Verification items for the finished model (mm, model axes). Face numbers are marked on the shaded views. A direction names the side the tool comes from. Coordinates: 2 decimals unless noted, no trailing zeros. Write each loop counter-clockwise with the first axis right and the second up, starting at its lowest first coordinate (ties: lowest second). Pieces come first, ordered by that corner, then holes. Notation, with made-up numbers: (18.25, 19.25) -> (30.25, 19.25) arc R20 ccw to (30.25, 24.25) -> close; hole circle Ø6 at (4, -37.75). An arc over 180 degrees is marked (long way). Use CSV: the item, a comma, the result in double quotes.
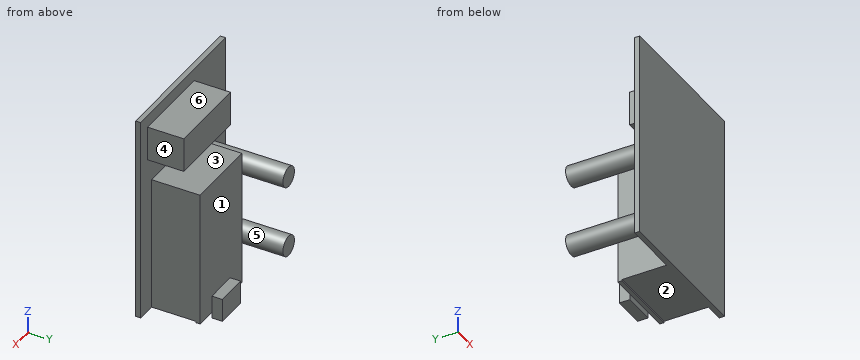
Autodesk Fusion 360 part; units mm, degrees
sketch "Sketch1" plane through (0, 0, 0) normal (0, 1, 0) x (1, 0, 0)
  line L0 (0, 0) -> (37, 0)
  line L1 (37, 0) -> (37, 51)
  line L2 (37, 51) -> (0, 51)
  line L3 (0, 51) -> (0, 0)
  line L4 (13.7, 3) -> (34, 3)
  line L5 (34, 3) -> (34, 11.5)
  line L6 (34, 11.5) -> (13.7, 11.5)
  line L7 (13.7, 11.5) -> (13.7, 3)
  line L8 (14, 17.75) -> (32.25, 17.75)
  line L9 (32.25, 17.75) -> (32.25, 51.35)
  line L10 (32.25, 51.35) -> (14, 51.35)
  line L11 (14, 51.35) -> (14, 17.75)
  line L12 (19.125, 47.15) -> (27.125, 47.15)
  line L13 (27.125, 47.15) -> (27.125, 52.85)
  line L14 (27.125, 52.85) -> (19.125, 52.85)
  line L15 (19.125, 52.85) -> (19.125, 47.15)
  circle A0 centre (9.5, 41.5) radius 2.5
  circle A1 centre (9.5, 23.5) radius 2.5
  dimension "d1" = 37
  dimension "d2" = 51
  dimension "d3" = 3
  dimension "d4" = 3
  dimension "d5" = 20.3
  dimension "d6" = 8.5
  dimension "d7" = 6.25
  dimension "d8" = 18.25
  dimension "d9" = 4.75
  dimension "d10" = 33.6
  dimension "d11" = 5.7
  dimension "d12" = 8
  dimension "d13" = 5.125
  dimension "d15" = 1.5
  dimension "d16" = 9.5
  dimension "d17" = 9.5
  dimension "d18" = 5
  dimension "d19" = 27.5
extrude "Extrude1" add sketch "Sketch1" against normal blind 1.25 contours L0 L1 L2 L3 L8 L9 L11 | L2 L8 L9 L11 L12 L13 L15 | L2 L12 L13 L15 | L4 L5 L6 L7 | A0 | A1
extrude "Extrude2" add sketch "Sketch1" along normal blind 9 contours L4 L5 L6 L7
extrude "Extrude3" add sketch "Sketch1" along normal blind 11 contours L2 L8 L9 L11 L12 L13 L15 | L2 L12 L13 L15
sketch "Sketch3" plane through (0, 11, 0) normal (0, 1, 0) x (-1, 0, 0)
  line L0 (-32.25, -51) -> (-14, -51)
  line L1 (-14, -51) -> (-14, -17.75)
  line L2 (-14, -17.75) -> (-32.25, -17.75)
  line L3 (-32.25, -17.75) -> (-32.25, -51)
  line L4 (-14, -17.75) -> (-32.25, -17.75)
  line L5 (-32.25, -17.75) -> (-32.25, -51.35)
  line L6 (-32.25, -51.35) -> (-14, -51.35)
  line L7 (-14, -51.35) -> (-14, -17.75)
  dimension "d26" = 33.6
  dimension "d27" = 18.25
extrude "Extrude4" add sketch "Sketch3" along normal blind 1
sketch "Sketch4" plane through (0, 12, 0) normal (0, 1, 0) x (-1, 0, 0)
  line L0 (-14, -51.35) -> (-14, -17.75)
  line L1 (-14, -17.75) -> (-32.25, -17.75)
  line L2 (-32.25, -17.75) -> (-32.25, -51.35)
  line L3 (-32.25, -51.35) -> (-14, -51.35)
  line L4 (-19.125, -47.15) -> (-27.125, -47.15)
  line L5 (-27.125, -47.15) -> (-27.125, -52.85)
  line L6 (-27.125, -52.85) -> (-19.125, -52.85)
  line L7 (-19.125, -52.85) -> (-19.125, -47.15)
  line L8 (-32.25, -51.35) -> (-14, -51.35)
  dimension "d30" = 5.125
  dimension "d31" = 8
  dimension "d32" = 5.7
  dimension "d33" = 1.5
extrude "Extrude5" add sketch "Sketch4" along normal blind 2.6 contours L3 L5 L6 L7 L8 | L3 L4 L5 L7 L8
extrude "Extrude6" add sketch "Sketch1" along normal blind 21 contours A0 | A1
sketch "Sketch6" plane through (0, -1.25, 0) normal (0, -1, 0) x (1, 0, 0)
  line L0 (0, 0) -> (0, -51)
  line L1 (0, -51) -> (37, -51)
  line L2 (37, -51) -> (37, 0)
  line L3 (37, 0) -> (0, 0)
  line L4 (4, -4) -> (33, -4)
  line L5 (33, -4) -> (33, -49)
  line L6 (33, -49) -> (4, -49)
  line L7 (4, -49) -> (4, -4)
  dimension "d38" = 2
  dimension "d39" = 4
  dimension "d41" = 4
  dimension "d42" = 4
  dimension "d45" = 29
  dimension "d46" = 45
extrude "Extrude7" [suppressed]
1) Cross-section at A-A (y = 7). Record the boundary of the cut face in (x, z).
Return value:
outline,"circle Ø5 at (9.5, -41.5); circle Ø5 at (9.5, -23.5); (13.7, -11.5) -> (34, -11.5) -> (34, -3) -> (13.7, -3) -> close; (14, -51) -> (32.25, -51) -> (32.25, -17.75) -> (14, -17.75) -> close"
2) Mould release check, pull along Z, two halves, no side actions. Record for the marked faces 1, 2 and 3: released by +Z, released by -Z, zero draft, split by the parting line, or undercut.
Return value:
face 1,"zero draft"
face 2,"released by -Z"
face 3,"undercut"
3) Gauge pin test, flat ends, axial feed: pin 1 (6 mm diameter, centred on y = 7.5, z = -36.5, fed in from -X); pin 2 (6 mm diameter, centred on x = 26.5, y = 6, fed in from +Z); pin 3 (2.5 mm diameter, centred on y = 4, z = -7.5, fed in from +X). Record the tip position at first contact, or that the pin passes through.
Return value:
pin 1,"x = 8"
pin 2,"z = -3"
pin 3,"x = 34"
4) Set-up check for the marked faces 4, 5 and 6: record each of +Z, -Z, +X, -X, +Y, -Y from which the full face is reachable in a straight line by a thin tool's end or side.
Return value:
face 4,"+Z, -Z, +X, +Y"
face 5,"+Y"
face 6,"+Z, +X, -X, +Y"
5) Scan lines: L1, parallel to Z at x = 19, y = 7; L2, parallel to Y at x = 3, z = -3; L3, parallel to Y at x = 31, z = -10.5. Record each from-to range of solid material in increasing order.
Return value:
L1,"-51 to -17.75, -11.5 to -3"
L2,"-1.25 to 0"
L3,"-1.25 to 9"
6) Cross-section at B-B (x = 9.5). Record the boundary of the cut face in (y, z), plus the area to 3 significant figures.
Return value:
outline,"(-1.25, -51) -> (0, -51) -> (0, -44) -> (21, -44) -> (21, -39) -> (0, -39) -> (0, -26) -> (21, -26) -> (21, -21) -> (0, -21) -> (0, 0) -> (-1.25, 0) -> close"
area,"274 mm2"
7) Cross-section at C-C (z = -23.5). Record the boundary of the cut face in (x, y).
Return value:
outline,"(0, -1.25) -> (37, -1.25) -> (37, 0) -> (32.25, 0) -> (32.25, 12) -> (14, 12) -> (14, 0) -> (12, 0) -> (12, 21) -> (7, 21) -> (7, 0) -> (0, 0) -> close"
8) Cross-section at D-D (y = 17.25). Record the boundary of the cut face in (x, z), plus the area to 3 significant figures.
Return value:
outline,"circle Ø5 at (9.5, -41.5); circle Ø5 at (9.5, -23.5)"
area,"39.3 mm2"
